from build123d import *

# Parameters (mm, degrees)
SKETCH1_R               = 32.5
SKETCH1_R_2             = 31.5
EXTRUDE_THIN1_DEPTH     = 40
SKETCH2_R               = 2
CUT_EXTRUDE1_DEPTH      = 61.930288035
CIRPATTERN1_START       = -32.500000066
CIRPATTERN1_OUTLINE_R   = 2
CIRPATTERN1_DEPTH       = 65.000000132
CIRPATTERN1_2_OUTLINE_R = 2
CIRPATTERN1_2_DEPTH     = 65.000000132
EXTRUDE_THIN2_START     = 2
SKETCH3_R               = 32.5
SKETCH3_R_2             = 24.5
EXTRUDE_THIN2_DEPTH     = 2
CHAMFER1_SIZE           = 1


# Read off the part's stored shape, not the designer's step: CirPattern1
with BuildPart() as part:
    # Sketch1 → Extrude-Thin1 (new body)
    with BuildSketch(Plane(origin=(0, 0, 0), x_dir=(0, 1, 0), z_dir=(0, 0, 1))):
        Circle(SKETCH1_R)
        Circle(SKETCH1_R_2, mode=Mode.SUBTRACT)
    extrude(amount=EXTRUDE_THIN1_DEPTH)

    # Sketch2 → Cut-Extrude1 (cut, symmetric)
    with BuildSketch(Plane(origin=(0, 0, 0), x_dir=(-1, 0, 0), z_dir=(0, 1, 0))):
        with Locations(Location((0, 17.085, 0), (0, 0, 90))):
            Circle(SKETCH2_R)
    extrude(amount=CUT_EXTRUDE1_DEPTH, both=True, mode=Mode.SUBTRACT)

    # CirPattern1 outline → CirPattern1 (cut)
    with BuildSketch(Plane(origin=(0, 0, 0), x_dir=(0.500000000000004, -0.8660254037844363, 0), z_dir=(0.8660254037844363, 0.5000000000000042, 0)).offset(CIRPATTERN1_START)):
        with Locations((0, -17.085)):
            Circle(CIRPATTERN1_OUTLINE_R)
    extrude(amount=CIRPATTERN1_DEPTH, mode=Mode.SUBTRACT)

    # CirPattern1 2 outline → CirPattern1 2 (cut)
    with BuildSketch(Plane(origin=(0, 0, 0), x_dir=(0.49999999999999767, 0.86602540378444, 0), z_dir=(0.8660254037844399, -0.49999999999999795, 0)).offset(CIRPATTERN1_START)):
        with Locations((0, 17.085)):
            Circle(CIRPATTERN1_2_OUTLINE_R)
    extrude(amount=CIRPATTERN1_2_DEPTH, mode=Mode.SUBTRACT)

    # Sketch3 → Extrude-Thin2 (add)
    with BuildSketch(Plane(origin=(0, 0, 0), x_dir=(1, 0, 0), z_dir=(0, 0, -1)).offset(EXTRUDE_THIN2_START)):
        Circle(SKETCH3_R)
        Circle(SKETCH3_R_2, mode=Mode.SUBTRACT)
    extrude(amount=-EXTRUDE_THIN2_DEPTH)

    # Chamfer1
    chamfer1_edges = [part.edges().sort_by_distance(p)[0] for p in [
        (0, -31.5, 40),
    ]]
    chamfer(chamfer1_edges, length=CHAMFER1_SIZE - 0.0001)  # a hair under: the kernel refuses the full size


solid = part.part
Model file for the job. Use its own axes, mm. A direction names the side the tool comes from. Give positions to 0.01 mm unless a question says otherwise; leave off trailing zeros. Loops run counter-clockwise (first coordinate to the right, second up) from the corner with the lowest first, then second, coordinate; pieces in that order, holes last. Notation, with made-up numbers: (58, 55.25) -> (117, 55.25) arc R11 cw to (117, 65.25) -> close; hole circle Ø2 at (55.5, -26.75). An arc over 180 degrees is marked (long way). Use a Markdown table: item, result. Add a question column.
(1) Tool access for faces 3 (the flat face through (16, 19, 0)), 4 (the cylindrical face through (-28.69, 14.257, 17.173)): list every direction of +Z, -Z, +X, -X, +Y, -Y with a clear straight run to the whole face (end or side of a thin tool).
(2) Slice it at C-C on z = 14. List the corners of the cut face in (x, y), and give its area (3 significant figures).
(3) Slice it at B-B on x = 0. Give the number of separate pieces and of enclosed holes in the cut face, and give its area (3 significant figures).
(4) Mould opens along Y. For faces 1 (the cylindrical face through (-0.77, 31.98, 18.93)), 2 (the cylindrical face through (-31.232, -4.101, 19.227)) say: +Y half, -Y half, draft (parallel to the pull), parting line (faces both ways), or undercut.
(5) Drop flat-ended pins along their axis: pin 1 Ø4 at (y, z) = (7.5, 12.5) entering from -X; pin 2 Ø5 at (x, z) = (-3, 6) entering from +Y; pin 3 Ø1.5 at (x, z) = (-9, 8.5) entering from +Y. Give the stop position or say it passes through.
(6) Wall check: line 1 along Y through (x, z) = (0.5, 6); line 2 along Y through (x, z) = (0, -1). Give the ranges that are in metal, low to high.
Filled sheet:
| question | item | result |
|---|---|---|
| 1 | face 3 | +Z |
| 1 | face 4 | none |
| 2 | outline | circle Ø65 at (0, 0); hole circle Ø63 at (0, 0) |
| 2 | area | 201 mm2 |
| 3 | separate pieces | 4 |
| 3 | enclosed holes | 0 |
| 3 | area | 103 mm2 |
| 4 | face 1 | draft |
| 4 | face 2 | undercut |
| 5 | pin 1 | x = -32.03 |
| 5 | pin 2 | y = 32.5 |
| 5 | pin 3 | y = 31.44 |
| 6 | line 1 | -32.5 to -31.5, 31.5 to 32.5 |
| 6 | line 2 | -32.5 to -24.5, 24.5 to 32.5 |
